Read the model definition and answer for the solid it produces. Units are mm, in the model's axes. A direction names the side the tool comes from. Coordinates: 2 decimals unless noted, no trailing zeros. Write each loop counter-clockwise with the first axis right and the second up, starting at its lowest first coordinate (ties: lowest second). Pieces come first, ordered by that corner, then holes.
(1) Section B-B on z = -60.2 is taken. Write down the section's boundary in (x, y).
(2) The mould has two halves that part along Z. Classify faces 6 (the flat face through (110, 10, -10)), 7 (the cylindrical face through (73.092, 10.601, -115.47)), 8 (the cylindrical face through (98.193, 15.07, -43.74)): +Z half, -Z half, draft (parallel to the pull), parting line (faces both ways), or undercut.
(3) Given pin 1 (4.5 mm diameter, centred on x = 54, z = -77.5, fed in from +Y); pin 2 (2 mm diameter, centred on x = 39.5, y = 10.5, fed in from -Z); pin 3 (3.5 mm diameter, centred on x = 110, y = 10, fed in from +Z), each flat-ended and moving along its own axis, determine where each tip first touches the part or whether it passes through.
(4) Section D-D on z = -43.48 is taken. Write down the section's boundary in (x, y), then the cut area to 3 significant figures.
(5) Section A-A on x = 145 is taken. Write down the section's boundary in (y, z).
(6) Section C-C on x = 110 is taken. Write down the section's boundary in (y, z).
(7) Which of the six approach directions +Z, -Z, +X, -X, +Y, -Y give full straight-line access (tool end or side, diameter ignored) to faces 1 (the flat face through (74, 12, 0)), 2 (the flat face through (96, 10, -77)), 3 (the flat face through (40, 10, -10)), 4 (the flat face through (40, 10, -110.4)), 5 (the cylindrical face through (143.8, 10.1, -106.8))?
(8) Find the intervals of material crossed by probe 1 along X at (y, z) = (15.25, -43.48); probe 2 along X at (y, z) = (10, -2); probe 3 along Z at (x, y) = (145, 4.5), in increasing order.
from build123d import *

# Parameters (mm, degrees)
SKETCH1_W                  = 150
SKETCH1_H                  = 120.4
BOSS_EXTRUDE2_DEPTH        = 20
SZKIC4_R                   = 2
WYTNIJ_WYCI_GNI_CIE2_DEPTH = 10
WYTNIJ_WYCI_GNI_CIE3_START = -10
SZKIC5_R                   = 2
WYTNIJ_WYCI_GNI_CIE3_DEPTH = 10
SZKIC1_R                   = 2
WYTNIJ_WYCI_GNI_CIE5_DEPTH = 10
SZKIC6_R                   = 2
WYTNIJ_WYCI_GNI_CIE6_DEPTH = 20


with BuildPart() as part:
    # Sketch1 → Boss-Extrude2 (new body)
    with BuildSketch(Plane(origin=(0, 0, 0), x_dir=(1, 0, 0), z_dir=(0, 1, 0))):
        with Locations((75, 60.2)):
            Rectangle(SKETCH1_W, SKETCH1_H)
    extrude(amount=BOSS_EXTRUDE2_DEPTH)

    # Szkic4 → Wytnij-wyciągnięcie2 (cut)
    with BuildSketch(Plane(origin=(0, 0, -120.4), x_dir=(-1, 0, 0), z_dir=(0, 0, -1))):
        with Locations((-40, 10)):
            Circle(SZKIC4_R)
        with Locations((-75, 10)):
            Circle(SZKIC4_R)
        with Locations((-110, 10)):
            Circle(SZKIC4_R)
    extrude(amount=-WYTNIJ_WYCI_GNI_CIE2_DEPTH, mode=Mode.SUBTRACT)

    # Szkic5 → Wytnij-wyciągnięcie3 (cut)
    with BuildSketch(Plane.XY.offset(WYTNIJ_WYCI_GNI_CIE3_START)):
        with Locations(Location((40, 10, 0), (0, 0, 180))):
            Circle(SZKIC5_R)
        with Locations(Location((75, 10, 0), (0, 0, 180))):
            Circle(SZKIC5_R)
        with Locations(Location((110, 10, 0), (0, 0, 180))):
            Circle(SZKIC5_R)
    extrude(amount=WYTNIJ_WYCI_GNI_CIE3_DEPTH, mode=Mode.SUBTRACT)

    # Szkic1 → Wytnij-wyciągnięcie5 (cut)
    with BuildSketch(Plane(origin=(0, 20, 0), x_dir=(1, 0, 0), z_dir=(0, 1, 0))):
        with Locations(Location((53.79, 76.92, 0), (0, 0, 270))):
            Circle(SZKIC1_R)
        with Locations(Location((96.21, 76.92, 0), (0, 0, 270))):
            Circle(SZKIC1_R)
        with Locations(Location((53.79, 43.48, 0), (0, 0, 270))):
            Circle(SZKIC1_R)
        with Locations(Location((96.21, 43.48, 0), (0, 0, 270))):
            Circle(SZKIC1_R)
    extrude(amount=-WYTNIJ_WYCI_GNI_CIE5_DEPTH, mode=Mode.SUBTRACT)

    # Szkic6 → Wytnij-wyciągnięcie6 (cut)
    with BuildSketch(Plane(origin=(0, 20, 0), x_dir=(1, 0, 0), z_dir=(0, 1, 0))):
        with Locations(Location((145, 105.2, 0), (0, 0, 270))):
            Circle(SZKIC6_R)
        with Locations(Location((145, 60.2, 0), (0, 0, 270))):
            Circle(SZKIC6_R)
        with Locations(Location((145, 15.2, 0), (0, 0, 270))):
            Circle(SZKIC6_R)
        with Locations(Location((5, 15.2, 0), (0, 0, 270))):
            Circle(SZKIC6_R)
        with Locations(Location((5, 60.2, 0), (0, 0, 270))):
            Circle(SZKIC6_R)
        with Locations(Location((5, 105.2, 0), (0, 0, 270))):
            Circle(SZKIC6_R)
    extrude(amount=-WYTNIJ_WYCI_GNI_CIE6_DEPTH, mode=Mode.SUBTRACT)


solid = part.part
Response:
1. outline: (0, 0) - (3, 0) - (3, 20) - (0, 20) - close; (7, 0) - (143, 0) - (143, 20) - (7, 20) - close; (147, 0) - (150, 0) - (150, 20) - (147, 20) - close
2. face 6: +Z half
2. face 7: draft
2. face 8: undercut
3. pin 1: stops at y = 20
3. pin 2: stops at z = -110.4
3. pin 3: stops at z = -10
4. outline: (0, 0) - (150, 0) - (150, 20) - (98.21, 20) - (98.21, 10) - (94.21, 10) - (94.21, 20) - (55.79, 20) - (55.79, 10) - (51.79, 10) - (51.79, 20) - (0, 20) - close
4. area: 2,920 mm2
5. outline: (0, -120.4) - (20, -120.4) - (20, -107.2) - (0, -107.2) - close; (0, -103.2) - (20, -103.2) - (20, -62.2) - (0, -62.2) - close; (0, -58.2) - (20, -58.2) - (20, -17.2) - (0, -17.2) - close; (0, -13.2) - (20, -13.2) - (20, 0) - (0, 0) - close
6. outline: (0, -120.4) - (8, -120.4) - (8, -110.4) - (12, -110.4) - (12, -120.4) - (20, -120.4) - (20, 0) - (12, 0) - (12, -10) - (8, -10) - (8, 0) - (0, 0) - close
7. face 1: +Z, +X, -X, +Y, -Y
7. face 2: +Y
7. face 3: +Z
7. face 4: -Z
7. face 5: +Y, -Y
8. probe 1: x = 0 to 51.79, 55.79 to 94.21, 98.21 to 150
8. probe 2: x = 0 to 38, 42 to 73, 77 to 108, 112 to 150
8. probe 3: z = -120.4 to -107.2, -103.2 to -62.2, -58.2 to -17.2, -13.2 to 0
